Can you work these out from the drawing? Everything is in mm from the part's minimum corner. A direction names the side the tool comes from. Coordinates: 2 decimals unless noted, no trailing zeros. Order: outer loops, then holes, each group sorted by start corner. A loop starts at its lowest first (then second) coordinate and runs counter-clockwise, first axis right, second up. Notation, with made-up numbers: (-11.75, 81.25) -> (42.25, 81.25) arc R18 cw to (42.25, 96.25) -> close; hole circle Ø8 at (-11.5, 79). An arc over 180 degrees is marked (long way). Use a Markdown table: item, result. Add a question column.
1) Thinking about a two-plate mould opening in X: for the marked faces 3, 4 and 5, which applies, +X half, -X half, draft (parallel to the pull), parting line (faces both ways), or undercut?
2) If we section it at A-A (y = 52): Write out the boundary of the cut face in (x, z) (3 decimals), plus the area to 3 significant figures.
3) If we section it at B-B (z = 78): Write out the boundary of the cut face in (x, y) (3 decimals).
4) Which directions (+Z, -Z, +X, -X, +Y, -Y) give clear straight access to the entire face, cutting with the end or side of a thin tool? Please do the marked faces 1 and 2.
5) If I drill on L1, parallel to X at y = 69, z = 16.5 (3 decimals); L2, parallel to Y at x = 104, z = 30 (3 decimals); L3, parallel to X at y = 71, z = 93.5, over which ranges is the centre line in solid material (lowest first)? Write a range as [from, to].
6) If we section it at C-C (x = 12.5): Write out the boundary of the cut face in (y, z) (3 decimals), plus the area to 3 significant figures.
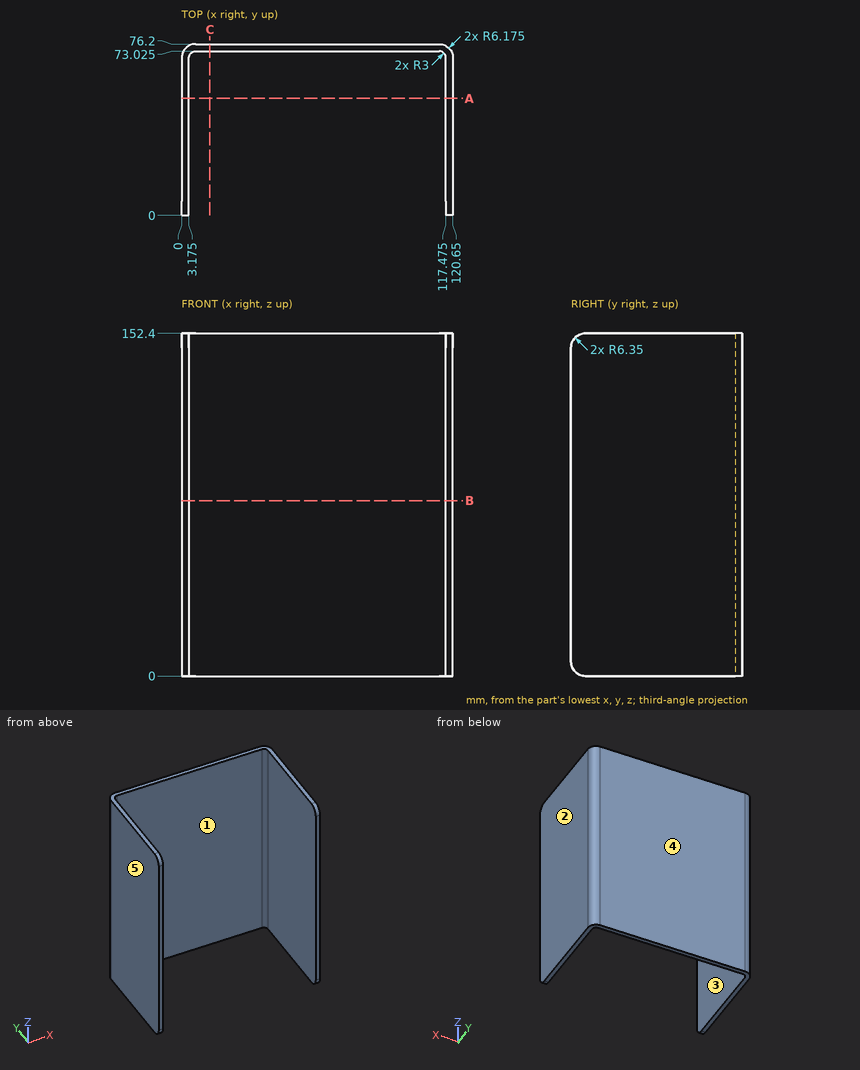
Answer sheet:
| question | item | result |
|---|---|---|
| 1 | face 3 | undercut |
| 1 | face 4 | draft |
| 1 | face 5 | -X half |
| 2 | outline | (0, 0) -> (3.175, 0) -> (3.175, 152.4) -> (0, 152.4) -> close; (117.475, 0) -> (120.65, 0) -> (120.65, 152.4) -> (117.475, 152.4) -> close |
| 2 | area | 968 mm2 |
| 3 | outline | (0, 0) -> (3.175, 0) -> (3.175, 70.025) arc R3 cw to (6.175, 73.025) -> (114.475, 73.025) arc R3 cw to (117.475, 70.025) -> (117.475, 0) -> (120.65, 0) -> (120.65, 70.025) arc R6.175 ccw to (114.475, 76.2) -> (6.175, 76.2) arc R6.175 ccw to (0, 70.025) -> close |
| 4 | face 1 | +Z, -Z, -Y |
| 4 | face 2 | +Z, -Z, +X, +Y, -Y |
| 5 | L1 | [0, 3.175], [117.475, 120.65] |
| 5 | L2 | [73.025, 76.2] |
| 5 | L3 | [0.08, 3.34], [117.31, 120.57] |
| 6 | outline | (73.025, 0) -> (76.2, 0) -> (76.2, 152.4) -> (73.025, 152.4) -> close |
| 6 | area | 484 mm2 |
